Can you work these out from the model? Positions are in its coordinate system, mm. Round coordinates to 2 decimals unless told otherwise and drop trailing zeros. Order: outer loops, then holes, each group sorted by start corner. A loop starts at its lowest first (then second) coordinate and runs counter-clockwise, first axis right, second up.
Q1. If we section it at A-A (z = 92): Please give me the cut outline in (x, y).
Q2. If we section it at B-B (y = -8.25): Please give me the cut outline in (x, z).
Q3. If I drill on line 1 (X direction, y = -5, z = 90.75); line 2 (Y direction, x = 145, z = 94.75); line 3 (X direction, y = -7.5, z = 31.5), over which ranges is the centre line in solid material (lowest first)?
Q4. Will this pin go through, and if not, where does the flat tip stop? P1, Ø2.5, axis at x = 145, y = -5, coming from the -Z side.
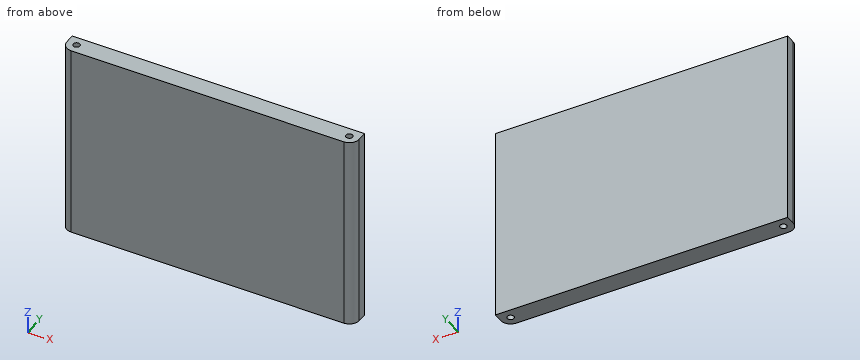
from build123d import *

# Parameters (mm, degrees)
F0_W     = 150
F0_H     = 100
F1_DEPTH = 10
F3_D     = 3.4
F3_DEPTH = 12
F3_TIP   = 1.0214630523
F4_D     = 3.4
F4_DEPTH = 12
F4_TIP   = 1.0214630523
F6_D     = 3.4
F6_DEPTH = 12
F6_TIP   = 1.0214630523
F7_D     = 3.4
F7_DEPTH = 12
F7_TIP   = 1.0214630523
F8_R     = 5
F9_R     = 5


with BuildPart() as f1:
    # F0 (on Front) → F1 (new body)
    with BuildSketch(Plane.XZ):
        with Locations((75, 50)):
            Rectangle(F0_W, F0_H)
    extrude(amount=F1_DEPTH)

    # F3
    with Locations(Plane.XY.offset(100)):
        with Locations((145, -5)):
            Hole(F3_D / 2, depth=F3_DEPTH)
            with Locations((0, 0, -(F3_DEPTH + F3_TIP / 2))):  # 118° drill point
                Cone(0, F3_D / 2, F3_TIP, mode=Mode.SUBTRACT)

    # F4
    with Locations(Plane.XY.offset(100)):
        with Locations((5, -5)):
            Hole(F4_D / 2, depth=F4_DEPTH)
            with Locations((0, 0, -(F4_DEPTH + F4_TIP / 2))):  # 118° drill point
                Cone(0, F4_D / 2, F4_TIP, mode=Mode.SUBTRACT)

    # F6
    with Locations(Plane(origin=(0, 0, 0), x_dir=(1, 0, 0), z_dir=(0, 0, -1))):
        with Locations((145, 5)):
            Hole(F6_D / 2, depth=F6_DEPTH)
            with Locations((0, 0, -(F6_DEPTH + F6_TIP / 2))):  # 118° drill point
                Cone(0, F6_D / 2, F6_TIP, mode=Mode.SUBTRACT)

    # F7
    with Locations(Plane(origin=(0, 0, 0), x_dir=(1, 0, 0), z_dir=(0, 0, -1))):
        with Locations((5, 5)):
            Hole(F7_D / 2, depth=F7_DEPTH)
            with Locations((0, 0, -(F7_DEPTH + F7_TIP / 2))):  # 118° drill point
                Cone(0, F7_D / 2, F7_TIP, mode=Mode.SUBTRACT)

    # F8
    f8_edges = [f1.edges().sort_by_distance(p)[0] for p in [
        (150, -10, 50),
    ]]
    fillet(f8_edges, radius=F8_R)

    # F9
    f9_edges = [f1.edges().sort_by_distance(p)[0] for p in [
        (0, -10, 50),
    ]]
    fillet(f9_edges, radius=F9_R)


solid = f1.part
Solution:
1. outline: (0, -5) arc R5 ccw to (5, -10) - (145, -10) arc R5 ccw to (150, -5) - (150, 0) - (0, 0) - close; hole circle Ø3.4 at (5, -5); hole circle Ø3.4 at (145, -5)
2. outline: (1.2, 0) - (148.8, 0) - (148.8, 100) - (1.2, 100) - close
3. line 1: x = 0 to 3.3, 6.7 to 143.3, 146.7 to 150
3. line 2: y = -10 to -6.7, -3.3 to 0
3. line 3: x = 0.67 to 149.33
4. P1: stops at z = 12.27
